```python
from build123d import *

# Parameters (mm, degrees)
F0_R     = 1.65
F0_R_2   = 5.25
F0_W     = 20
F0_H     = 40
F0_R_3   = 2.65
F1_DEPTH = 5
F2_W     = 6
F2_H     = 28.0157411588
F3_DEPTH = 6
F5_DEPTH = 20
F6_R     = 2.65
F7_DEPTH = 25
F9_DEPTH = 6


with BuildPart() as f1:
    # F0 (on Top) → F1 (new body)
    with BuildSketch(Plane.XY):
        Polygon((-69.0715216601, -47.4452535896), (-69.0715216601, -47.4295124308), (-69.0715216601, -7.4295124308), (-99.0715216601, -7.4295124308), (-104.0715216601, -7.4295124308), (-104.0715216601, -17.4295124308), (-104.0715216601, -37.4295124308), (-104.0715216601, -47.4452535896), (-99.1652225519, -47.4452535896), align=None)
        with Locations((-99.7324526625, -33.0822869872)):
            Circle(F0_R, mode=Mode.SUBTRACT)
        with Locations((-88.4105906576, -33.0822869872)):
            Circle(F0_R, mode=Mode.SUBTRACT)
        with Locations((-94.0715216601, -27.4295124308)):
            Circle(F0_R_2, mode=Mode.SUBTRACT)
        with Locations((-99.7324526625, -21.7767378744)):
            Circle(F0_R, mode=Mode.SUBTRACT)
        with Locations((-88.4105906576, -21.7767378744)):
            Circle(F0_R, mode=Mode.SUBTRACT)
        with Locations((-59.0715216601, -27.4295124308)):
            Rectangle(F0_W, F0_H)
        with Locations((-59.0715216601, -40.4295124308)):
            Circle(F0_R_3, mode=Mode.SUBTRACT)
        with Locations((-58.7309271957, -14.4295124308)):
            Circle(F0_R_3, mode=Mode.SUBTRACT)
    extrude(amount=F1_DEPTH)

    # F2 (on face) → F3 (join)
    with BuildSketch(Plane.XY.offset(5)):
        Polygon((-64.0715216601, -7.4295124308), (-104.0715216601, -7.4295124308), (-104.0715216601, -13.4295124308), (-70.0715216601, -13.4295124308), (-64.0715216601, -13.4295124308), align=None)
        with Locations((-67.0715216601, -27.4373830102)):
            Rectangle(F2_W, F2_H)
        Polygon((-70.0715216601, -41.4452535896), (-104.0715216601, -41.4452535896), (-104.0715216601, -47.4452535896), (-69.0715216601, -47.4452535896), (-69.0715216601, -47.4295124308), (-64.0715216601, -47.4295124308), (-64.0715216601, -41.4452535896), align=None)
    extrude(amount=F3_DEPTH)

    # F4 (on face) → F5 (join)
    with BuildSketch(Plane.XY):
        Polygon((-76.0715216601, -47.4452535896), (-69.0715216601, -47.4452535896), (-69.0715216601, -47.4295124308), (-69.0715216601, -7.4452535896), (-76.0715216601, -7.4452535896), align=None)
    extrude(amount=-F5_DEPTH)

    # F6 (on face) → F7 (cut)
    with BuildSketch(Plane(origin=(-76.0715216601, 0, 0), x_dir=(0, -1, 0), z_dir=(-1, 0, 0))):
        with Locations((27.4452535896, -10)):
            Circle(F6_R)
    extrude(amount=-F7_DEPTH, mode=Mode.SUBTRACT)

    # F8 (on face) → F9 (join)
    with BuildSketch(Plane.XY):
        Polygon((-99.1652225519, -47.4452535896), (-76.0715216601, -47.4452535896), (-76.0715216601, -40.4452535896), (-104.0715216601, -40.4452535896), (-104.0715216601, -47.4452535896), align=None)
        Polygon((-76.0715216601, -14.4295124308), (-76.0715216601, -7.4295124308), (-99.0715216601, -7.4295124308), (-104.0715216601, -7.4295124308), (-104.0715216601, -14.4295124308), align=None)
    extrude(amount=-F9_DEPTH)


solid = f1.part
```
Source: CAD feature listing. Evaluate the final solid. Frame: model axes, mm. A direction names the side the tool comes from. Coordinates: 2 decimals unless noted, no trailing zeros. Loops run counter-clockwise (first coordinate to the right, second up) from the corner with the lowest first, then second, coordinate; pieces in that order, holes last. Notation, with made-up numbers: M -25.5,80 L 33.5,80 A9 ccw 33.5,93 Z; hole C 48.5,-13.5 d1. An arc over 180 degrees is marked long. Put each result on its own line as item: value. Start each with the question number.
1) Pull-direction query (X, two-part tool) for faces 1 (the face through (-73, -27, -20)), 2 (the face through (-59.4, -37.8, 2.5)), 3 (the face through (-64.072, -28, 8)); classes: pulls with the +X half, pulls with the -X half, needs draft (parallel to the pull), parting line crosses it, or undercut.
2) Cut plane D-D on y = -10.5. Return the cut outline in (x, z).
3) Ray query, L1, parallel to Y at x = -98.5, z = -5; L2, parallel to X at y = -10, z = -9; L3, parallel to Z at x = -80.5, y = -11. Return the intervals inside material, ascending. Write a range as from..to.
4) Contact query for flat-ended pins moving along their axis: pin 1 Ø3.5 at (x, z) = (-62.5, 3.5) entering from -Y; pin 2 Ø16 at (y, z) = (-22, -11) entering from -X; pin 3 Ø5 at (y, z) = (-23.5, -3) entering from +X; pin 4 Ø2 at (x, y) = (-88.41, -33.08) entering from -Z. Output: stop coordinate, or through.
5) Cut plane C-C on z = 3.5. Give the number of separate pieces and of enclosed holes in the cut face, then the cut area to 3 significant figures.
6) Reachability of faces 4 (the face through (-72.62, -28.67, -12.35)), 5 (the face through (-57, -27, 5)), 6 (the face through (-90, -11, -6)) from +Z, -Z, +X, -X, +Y, -Y: full face, straight path, thin tool, end or side. Return the list, or none.
7) Cut plane A-A on z = -10. Return the cut outline in (x, y).
The answers:
1. face 1: needs draft
1. face 2: undercut
1. face 3: pulls with the +X half
2. outline: M -104.07,-6 L -76.07,-6 L -76.07,-20 L -69.07,-20 L -69.07,0 L -49.07,0 L -49.07,5 L -64.07,5 L -64.07,11 L -104.07,11 Z
3. L1: y = -47.45..-40.45, -14.43..-7.43
3. L2: x = -76.07..-69.07
3. L3: z = -6..11
4. pin 1: stops at y = -47.43
4. pin 2: stops at x = -76.07
4. pin 3: stops at x = -69.07
4. pin 4: passes through
5. separate pieces: 1
5. enclosed holes: 7
5. area: 2,040 mm²
6. face 4: +X, -X
6. face 5: +Z, +X, +Y, -Y
6. face 6: -Z, -X, +Y, -Y
7. outline: M -76.07,-47.45 L -69.07,-47.45 L -69.07,-30.1 L -76.07,-30.1 Z; M -76.07,-24.8 L -69.07,-24.8 L -69.07,-7.45 L -76.07,-7.45 Z
